```python
from build123d import *

# Parameters (mm, degrees)
BOSS_EXTRU_1_DEPTH      = 5
BOSS_EXTRU_1_DEPTH_BACK = 5
BOSS_EXTRU_2_DEPTH      = 120
BOSS_EXTRU_2_DEPTH_BACK = 120
ESQUISSE2_W             = 20
ESQUISSE2_H             = 20
ESQUISSE2_W_2           = 10
ESQUISSE2_H_2           = 10
ESQUISSE3_R             = 4.351117742
ENL_V_MAT_EXTRU_1_DEPTH = 120
ESQUISSE4_R             = 10
BOSS_EXTRU_3_DEPTH      = 20


with BuildPart() as part:
    # Esquisse1 → Boss.-Extru.1 (new, two sides: drawn at the far end of the back side and taken through both)
    with BuildSketch(Plane.XY.offset(-BOSS_EXTRU_1_DEPTH_BACK)):
        with BuildLine():
            Line((-100, 0), (-80, 0))
            ThreePointArc((-80, 0), (0, -80), (80, 0))
            Line((80, 0), (100, 0))
            ThreePointArc((100, 0), (0, -100), (-100, 0))
        make_face()
    extrude(amount=BOSS_EXTRU_1_DEPTH + BOSS_EXTRU_1_DEPTH_BACK)

    # Esquisse2 → Boss.-Extru.2 (add, two sides: drawn at the far end of the back side and taken through both)
    with BuildSketch(Plane(origin=(0, 0, 0), x_dir=(0, 0, -1), z_dir=(1, 0, 0)).offset(-BOSS_EXTRU_2_DEPTH_BACK)):
        with Locations((0, 10)):
            Rectangle(ESQUISSE2_W, ESQUISSE2_H)
        with Locations((0, 10)):
            Rectangle(ESQUISSE2_W_2, ESQUISSE2_H_2, mode=Mode.SUBTRACT)
    extrude(amount=BOSS_EXTRU_2_DEPTH + BOSS_EXTRU_2_DEPTH_BACK)

    # Esquisse3 → Enl_v. mat.-Extru.1 (cut)
    with BuildSketch(Plane(origin=(0, 0, -10), x_dir=(-1, 0, 0), z_dir=(0, 0, -1))):
        with Locations(Location((0, 10, 0), (0, 0, 180))):
            Circle(ESQUISSE3_R)
    extrude(amount=-ENL_V_MAT_EXTRU_1_DEPTH, mode=Mode.SUBTRACT)

    # Esquisse4 → Boss.-Extru.3 (add)
    with BuildSketch(Plane(origin=(0, 20, 0), x_dir=(1, 0, 0), z_dir=(0, 1, 0))):
        with Locations(Location((-80, 0, 0), (0, 0, 270))):
            Circle(ESQUISSE4_R)
        with Locations(Location((80, 0, 0), (0, 0, 270))):
            Circle(ESQUISSE4_R)
    extrude(amount=BOSS_EXTRU_3_DEPTH)


solid = part.part
```
Input: part model. Units: mm. Frame: model coordinates. A direction names the side the tool comes from. Give positions to 0.01 mm unless a question says otherwise; leave off trailing zeros. Loops run counter-clockwise (first coordinate to the right, second up) from the corner with the lowest first, then second, coordinate; pieces in that order, holes last.
1) Contact query for flat-ended pins moving along their axis: pin 1 (5 mm diameter, centred on y = -48, z = 4, fed in from +X); pin 2 (11.5 mm diameter, centred on x = 0, y = 10, fed in from -Z); pin 3 (3 mm diameter, centred on x = 45.5, z = 0, fed in from -Y); pin 4 (2 mm diameter, centred on x = -54.5, z = 3.5, fed in from +Y). Output: stop coordinate, or through.
A:
pin 1: stops at x = 89.05
pin 2: stops at z = -10
pin 3: stops at y = -89.8
pin 4: stops at y = 20
2) Mould query, pull axis Z, two halves, no side actions, for faces 1 (the flat face through (0, -83, -5)), 2 (the cylindrical face through (2.199, -99.976, -0.07)), 3 (the flat face through (-1.7, 5.5, -5)). Classes: released by +Z, released by -Z, zero draft, split by the parting line, or undercut.
A:
face 1: released by -Z
face 2: zero draft
face 3: undercut
3) Reachability of faces 4 (the cylindrical face through (-0.566, 5.686, -7.535)), 5 (the flat face through (80, 40, 0)), 6 (the cylindrical face through (-70.085, 29.86, -1.302)), 7 (the flat face through (0, -83, 5)), 8 (the flat face through (-2, 5, 0)) from +Z, -Z, +X, -X, +Y, -Y: full face, straight path, thin tool, end or side. Return the list, or none.
A:
face 4: +Z, -Z
face 5: +Z, -Z, +X, -X, +Y
face 6: +Y
face 7: +Z, +X, -X, -Y
face 8: +X, -X
4) Section query D-D on x = -74. Return the cut outline in (y, z).
A:
outline: (-67.26, -5) - (-30.4, -5) - (-30.4, 5) - (-67.26, 5) - close; (0, -10) - (20, -10) - (20, -8) - (40, -8) - (40, 8) - (20, 8) - (20, 10) - (0, 10) - close; hole (5, -5) - (15, -5) - (15, 5) - (5, 5) - close
5) Line query: L1, parallel to Y at x = 0, z = -8.7; L2, parallel to Y at x = -5.5, z = 1.25; L3, parallel to Y at x = -60, z = -2. Output: solid intervals per line, ascending.
A:
L1: y = 0 to 5.65, 14.35 to 20
L2: y = -99.85 to -79.81, 0 to 5, 15 to 20
L3: y = -80 to -52.92, 0 to 5, 15 to 20
6) Section query C-C on y = -44.5. Return the cut outline in (x, z).
A:
outline: (-89.55, -5) - (-66.48, -5) - (-66.48, 5) - (-89.55, 5) - close; (66.48, -5) - (89.55, -5) - (89.55, 5) - (66.48, 5) - close
7) Section query B-B on x = 65. Return the cut outline in (y, z), and give its area (3 significant figures).
A:
outline: (-75.99, -5) - (-46.64, -5) - (-46.64, 5) - (-75.99, 5) - close; (0, -10) - (20, -10) - (20, 10) - (0, 10) - close; hole (5, -5) - (15, -5) - (15, 5) - (5, 5) - close
area: 594 mm2
8) Section query A-A on z = 0. Return the cut outline in (x, y).
A:
outline: (-120, 0) - (-100, 0) arc R100 ccw to (100, 0) - (120, 0) - (120, 5) - (-120, 5) - close; (-120, 15) - (120, 15) - (120, 20) - (90, 20) - (90, 40) - (70, 40) - (70, 20) - (-70, 20) - (-70, 40) - (-90, 40) - (-90, 20) - (-120, 20) - close; hole (-80, 0) arc R80 ccw to (80, 0) - close
